Geometry check sheet. Reference: the model listing, model coordinates, mm. A direction names the side the tool comes from. Round coordinates to 2 decimals unless told otherwise and drop trailing zeros. Loops run counter-clockwise (first coordinate to the right, second up) from the corner with the lowest first, then second, coordinate; pieces in that order, holes last. Notation, with made-up numbers: (-13, 63.5) -> (9, 63.5) arc R24 cw to (9, 73.5) -> close; hole circle Ø6 at (-31, 30). An arc over 180 degrees is marked (long way). Use one line per item in the form item = value.
from build123d import *

# Parameters (mm, degrees)
F0_W     = 276.8
F0_H     = 12.5
F4_DEPTH = 4
F6_D     = 8
F6_DEPTH = 25
F6_TIP   = 2.4034424761
F8_DEPTH = 4


with BuildPart() as f1:
    # F0 (on Front) → F1 (revolve)
    with BuildSketch(Plane.XZ):
        with Locations((138.4, 6.25)):
            Rectangle(F0_W, F0_H)
    revolve(axis=Axis((138.4, 0, 0), (-1, 0, 0)))

    # F3 (on offset) → F4 (cut)
    with BuildSketch(Plane.XY.offset(12.5)):
        with BuildLine():
            Line((0, 4), (0, 0))
            Line((0, 0), (0, -4))
            Line((0, -4), (88, -4))
            ThreePointArc((88, -4), (90.8284271247, -2.8284271247), (92, 0))
            ThreePointArc((92, 0), (90.8284271247, 2.8284271247), (88, 4))
            Line((88, 4), (0, 4))
        make_face()
    extrude(amount=-F4_DEPTH, mode=Mode.SUBTRACT)

    # F6
    with Locations(Plane(origin=(0, 0, 0), x_dir=(0, -1, 0), z_dir=(-1, 0, 0))):
        with Locations((0, 0)):
            Hole(F6_D / 2, depth=F6_DEPTH)
            with Locations((0, 0, -(F6_DEPTH + F6_TIP / 2))):  # 118° drill point
                Cone(0, F6_D / 2, F6_TIP, mode=Mode.SUBTRACT)

    # F7 (on offset) → F8 (cut)
    with BuildSketch(Plane.XY.offset(12.5)):
        with BuildLine():
            ThreePointArc((208.5, 0), (207.3284271247, 2.8284271247), (204.5, 4))
            Line((204.5, 4), (162.5, 4))
            ThreePointArc((162.5, 4), (159.6715728753, 2.8284271247), (158.5, 0))
            ThreePointArc((158.5, 0), (159.6715728753, -2.8284271247), (162.5, -4))
            Line((162.5, -4), (204.5, -4))
            ThreePointArc((204.5, -4), (207.3284271247, -2.8284271247), (208.5, 0))
        make_face()
    extrude(amount=-F8_DEPTH, mode=Mode.SUBTRACT)


solid = f1.part
1. Gauge pin test, flat ends, axial feed: pin 1 (6.5 mm diameter, centred on x = 194, y = -2, fed in from +Z); pin 2 (8 mm diameter, centred on x = 219, z = 9, fed in from +Y); pin 3 (1.5 mm diameter, centred on x = 150, z = -8.5, fed in from -Y). Record the tip position at first contact, or that the pin passes through.
Return value:
pin_1 = 11.84
pin_2 = 11.46
pin_3 = -9.81
2. Section check C-C (z = -8.25). Record the boundary of the cut face in (x, y).
Return value:
outline = (0, -9.39) -> (276.8, -9.39) -> (276.8, 9.39) -> (0, 9.39) -> close
3. Mould release check, pull along X, two halves, no side actions. Record for faces 1 (the conical face through (26.986, 0.151, -0.678)), 2 (the cylindrical face through (12.675, -0.867, -3.905)), 3 (the flat face through (183, 0, 8.5)), 4 (the flat face through (276.8, 0, 0)): released by +X, released by -X, zero draft, split by the parting line, or undercut.
Return value:
face_1 = released by -X
face_2 = zero draft
face_3 = undercut
face_4 = released by +X
4. Tool access check on faces 5 (the flat face through (45, 0, 8.5)), 6 (the flat face through (0, 3, -3)). Record the directions out of +Z, -Z, +X, -X, +Y, -Y that give a thin tool (end or side, any length) a straight path to the whole face; none if there is none.
Return value:
face_5 = +Z, -X
face_6 = +Z, -Z, -X, +Y, -Y
5. Section check A-A (x = 211.5). Record the boundary of the cut face in (y, z).
Return value:
outline = circle Ø25 at (0, 0)
6. Section check B-B (y = 10.25). Record the boundary of the cut face in (x, z).
Return value:
outline = (0, -7.15) -> (276.8, -7.15) -> (276.8, 7.15) -> (0, 7.15) -> close
7. Material ranges on line 1 along Y through (x, z) = (14.75, 0); line 2 along Y through (x, z) = (72, 9.75); line 3 along Z through (x, y) = (30.5, 1), recorded low to high.
Return value:
line_1 = -12.5 to -4, 4 to 12.5
line_2 = -7.82 to -4, 4 to 7.82
line_3 = -12.46 to 8.5
